from build123d import *

# Parameters (mm, degrees)
BOSS_EXTRUDE1_DEPTH = 10
SKETCH2_R           = 1.75
CUT_EXTRUDE1_DEPTH  = 10
SKETCH3_R           = 1.25
SKETCH3_R_2         = 1.8
CUT_EXTRUDE2_DEPTH  = 40.143965052
CHAMFER1_SIZE       = 0.25
SKETCH4_W           = 13.022509218
SKETCH4_H           = 4.5
CUT_EXTRUDE3_DEPTH  = 40.143965052


with BuildPart() as part:
    # Sketch1 → Boss-Extrude1 (new body)
    with BuildSketch(Plane.XY):
        Polygon((0, 0), (0, 36.5), (12.5, 36.5), (12.5, 34), (2.5, 34), (2.5, 0), align=None)
    extrude(amount=BOSS_EXTRUDE1_DEPTH)

    # Sketch2 → Cut-Extrude1 (cut)
    with BuildSketch(Plane.XZ.offset(-34)):
        with Locations((7.5, 5)):
            Circle(SKETCH2_R)
    extrude(amount=-CUT_EXTRUDE1_DEPTH, mode=Mode.SUBTRACT)

    # Sketch3 → Cut-Extrude2 (cut, through all)
    with BuildSketch(Plane(origin=(2.5, 0, 0), x_dir=(0, 0, -1), z_dir=(1, 0, 0))):
        with Locations(Location((-3.25, 7.15, 0), (0, 0, 90))):
            Circle(SKETCH3_R)
        with Locations(Location((-3.25, 16.85, 0), (0, 0, 270))):
            Circle(SKETCH3_R)
        with Locations(Location((-5, 29, 0), (0, 0, 90))):
            Circle(SKETCH3_R_2)
    extrude(amount=-CUT_EXTRUDE2_DEPTH, mode=Mode.SUBTRACT)

    # Chamfer1
    chamfer1_edges = [part.edges().sort_by_distance(p)[0] for p in [
        (0, 0, 5),
        (0, 36.5, 5),
        (12.5, 36.5, 5),
        (2.5, 0, 5),
        (7.5, 34, 10),
        (12.5, 35.25, 10),
        (5.75, 36.5, 5),
        (6.25, 36.5, 10),
        (5.75, 34, 5),
        (0, 18.25, 10),
        (0, 5.9, 3.25),
        (0, 18.1, 3.25),
        (0, 27.2, 5),
        (1.25, 0, 10),
        (0, 18.25, 0),
        (6.25, 36.5, 0),
        (12.5, 35.25, 0),
        (7.5, 34, 0),
        (2.5, 17, 0),
        (1.25, 0, 0),
        (2.5, 17, 10),
    ]]
    chamfer(chamfer1_edges, length=CHAMFER1_SIZE)

    # Sketch4 → Cut-Extrude3 (cut, through all)
    with BuildSketch(Plane(origin=(2.5, 0, 0), x_dir=(0, 0, -1), z_dir=(1, 0, 0))):
        with Locations((-6.511254609, 2.25)):
            Rectangle(SKETCH4_W, SKETCH4_H)
    extrude(amount=-CUT_EXTRUDE3_DEPTH, mode=Mode.SUBTRACT)


solid = part.part
Model file for the job. Use its own axes, mm. A direction names the side the tool comes from. Give positions to 0.01 mm unless a question says otherwise; leave off trailing zeros. Loops run counter-clockwise (first coordinate to the right, second up) from the corner with the lowest first, then second, coordinate; pieces in that order, holes last. Notation, with made-up numbers: (10.25, 29.5) -> (25.25, 29.5) arc R23 cw to (25.25, 66.5) -> close; hole circle Ø4 at (66.5, 42.25). An arc over 180 degrees is marked (long way). Use a Markdown table: item, result. Add a question column.
(1) Slice it at C-C on y = 26.5. List the corners of the cut face in (x, z).
(2) Wall check: line 1 along Z through (x, y) = (0.85, 29); line 2 along X through (y, z) = (32, 1.25); line 3 along Z through (x, y) = (1.2, 7.15). Give the ranges that are in metal, low to high.
(3) Slice it at D-D on z = 2.5. Give the number of separate pieces and of enclosed holes in the cut face, and give its area (3 significant figures).
(4) Slice it at B-B on z = 7.5. List the corners of the cut face in (x, y), and give its area (3 significant figures).
(5) Mould opens along Z. For faces 1 (the cylindrical face through (1.391, 30.663, 4.311)), 2 (the cylindrical face through (8.31, 35.24, 3.45)), 3 (the flat face through (2, 25, 10)), 4 (the flat face through (5, 36.5, 5)) say: +Z half, -Z half, draft (parallel to the pull), parting line (faces both ways), or undercut.
(6) Drop flat-ended pins along their axis: pin 1 Ø3 at (x, z) = (7.5, 5) entering from -Y; pin 2 Ø1 at (y, z) = (14, 3.5) entering from +X. Give the stop position or say it passes through.
(7) Tool access for faces 5 (the flat face through (7.6, 34, 2.8)), 6 (the cylindrical face through (1.4, 5.9, 3.3)): list every direction of +Z, -Z, +X, -X, +Y, -Y with a clear straight run to the whole face (end or side of a thin tool).
(8) Slice it at A-A on y = 7.15. List the corners of the cut face in (x, z).
Filled sheet:
| question | item | result |
|---|---|---|
| 1 | outline | (0, 0.25) -> (0.25, 0) -> (2.25, 0) -> (2.5, 0.25) -> (2.5, 9.75) -> (2.25, 10) -> (0.25, 10) -> (0, 9.75) -> close |
| 2 | line 1 | 0 to 3.2, 6.8 to 10 |
| 2 | line 2 | 0 to 2.5 |
| 2 | line 3 | 0 to 2, 4.5 to 10 |
| 3 | separate pieces | 3 |
| 3 | enclosed holes | 0 |
| 3 | area | 94.8 mm2 |
| 4 | outline | (0, 4.5) -> (2.5, 4.5) -> (2.5, 34) -> (12.5, 34) -> (12.5, 36.25) -> (12.25, 36.5) -> (0.25, 36.5) -> (0, 36.25) -> close |
| 4 | area | 105 mm2 |
| 5 | face 1 | undercut |
| 5 | face 2 | undercut |
| 5 | face 3 | +Z half |
| 5 | face 4 | draft |
| 6 | pin 1 | through |
| 6 | pin 2 | x = 2.5 |
| 7 | face 5 | +Z, -Z, +X, -Y |
| 7 | face 6 | +X, -X |
| 8 | outline | (0, 0.25) -> (0.25, 0) -> (2.25, 0) -> (2.5, 0.25) -> (2.5, 2) -> (0.25, 2) -> (0, 1.75) -> close; (0, 4.75) -> (0.25, 4.5) -> (2.5, 4.5) -> (2.5, 9.75) -> (2.25, 10) -> (0.25, 10) -> (0, 9.75) -> close |
